The figure shows three views and two pictorial views of one solid part (mm, origin at its lowest corner). Answer the questions. A direction names the side the tool comes from. Give positions to 0.01 mm unless a question says otherwise; leave off trailing zeros. Write each loop counter-clockwise with the first axis right and the second up, starting at its lowest first coordinate (ties: lowest second). Pieces come first, ordered by that corner, then holes. Notation, with made-up numbers: (69, 85) -> (74, 85) arc R18 ccw to (74, 92) -> close; hole circle Ø8 at (84, -22.5). An arc over 180 degrees is marked (long way). Write item = value, one per line. Start each with the question number.
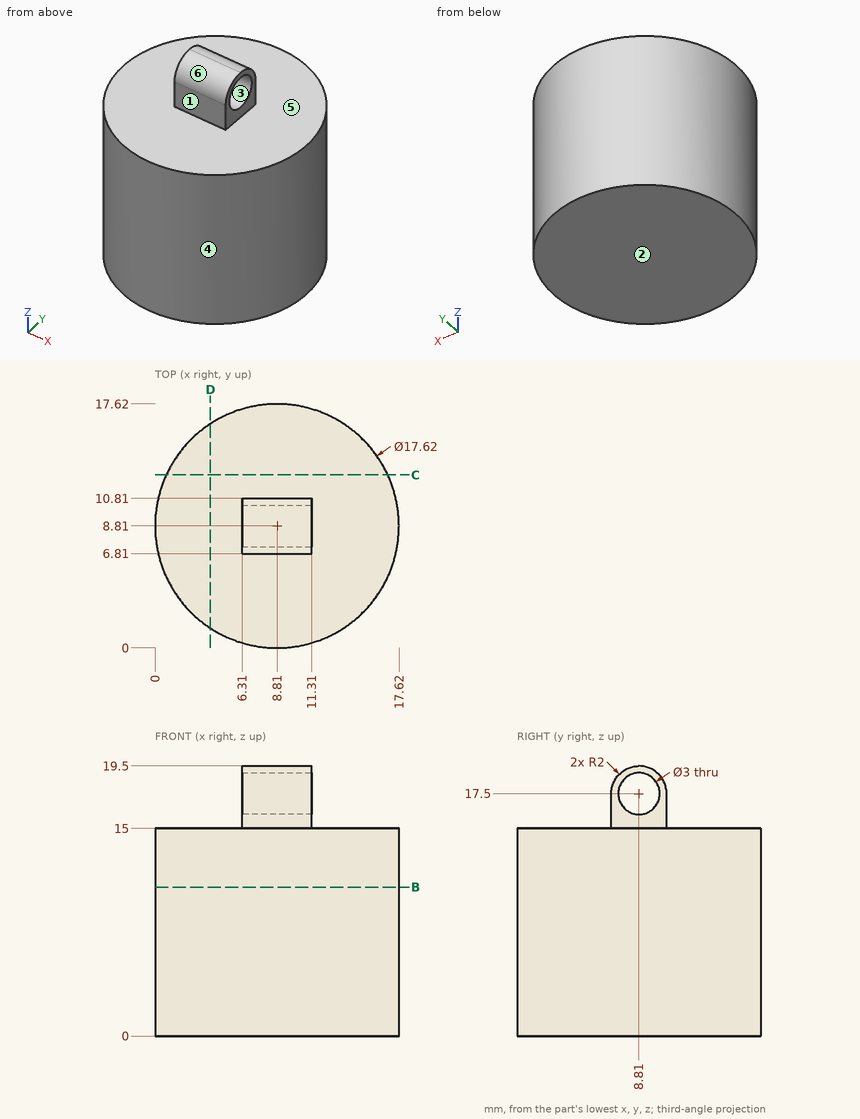
(1) Each of these flat-tipped pins is pushed along its axis until it touches: pin 1 (1.2 mm diameter, centred on y = 9.5, z = 17.5, fed in from -X); pin 2 (0.8 mm diameter, centred on x = 9, z = 16, fed in from +Y); pin 3 (4 mm diameter, centred on x = 15.5, y = 7.5, fed in from +Z); pin 4 (5 mm diameter, centred on x = 3.5, z = 3, fed in from +Y). Where does it stop, or does it pass through?
(2) For the marked faces 1 and 2, determine the directions among +Z, -Z, +X, -X, +Y, -Y from which every point of the face is accessible in a straight line to the end or side of a thin tool.
(3) A cutting plane is placed at C-C, the plane y = 12.5. Write down the section's boundary in (x, z).
(4) A cutting plane is placed at D-D, the plane x = 4. Write down the section's boundary in (y, z), then the cut area to 3 significant figures.
(5) A cutting plane is placed at B-B, the plane z = 10.75. Write down the section's boundary in (x, y).
(6) Determine the mould class of the marked faces 3, 4, 5 and 6 for opening direction Y: pulls with the +Y half, pulls with the -Y half, needs draft (parallel to the pull), parting line crosses it, or undercut.
(7) Find the intervals of material crossed by line 1 along Y through (x, z) = (9.7, 17.5); line 2 along X through (y, z) = (8.5, 10.75); line 3 along Z through (x, y) = (15.25, 9.5), in increasing order.
Results list:
q1.pin_1 = through
q1.pin_2 = 10.81
q1.pin_3 = 15
q1.pin_4 = 17.16
q2.face_1 = +Z, +X, -X, -Y
q2.face_2 = -Z, +X, -X, +Y, -Y
q3.outline = (0.81, 0) -> (16.81, 0) -> (16.81, 15) -> (0.81, 15) -> close
q4.outline = (1.43, 0) -> (16.19, 0) -> (16.19, 15) -> (1.43, 15) -> close
q4.area = 221 mm²
q5.outline = circle Ø17.62 at (8.81, 8.81)
q6.face_3 = undercut
q6.face_4 = parting line crosses it
q6.face_5 = needs draft
q6.face_6 = pulls with the -Y half
q7.line_1 = 6.81 to 7.31, 10.31 to 10.81
q7.line_2 = 0.01 to 17.61
q7.line_3 = 0 to 15
